Source: CAD feature listing. Evaluate the final solid. Frame: model axes, mm. Face numbers are marked on the shaded views. A direction names the side the tool comes from. Coordinates: 2 decimals unless noted, no trailing zeros. Write item = value, one per line. Start each with the question number.
1. Pull-direction query (Y, two-part tool) for the marked faces 1, 2 and 3; classes: pulls with the +Y half, pulls with the -Y half, needs draft (parallel to the pull), parting line crosses it, or undercut.
2. Pin query (flat end, axial travel): pin 1 Ø6 at (x, z) = (29.5, 2.5) entering from -Y; pin 2 Ø8 at (x, z) = (13, 4) entering from +Y; pin 3 Ø12 at (y, z) = (-34.5, 7) entering from -X. Return the tip coordinate at first contact, or that it passes through.
3. Section query A-A (z = 0.5). Give the number of separate pieces and of enclosed holes in the cut face, then the cut area to 3 significant figures.
4. Access query for the marked faces 4, 5 and 6. Directions: +Z, -Z, +X, -X, +Y, -Y. A direction counts if a zero-diameter tool reaches every point of the face in a straight line with its end or side. Return the directions, or none.
5. Line query: line 1 along X through (y, z) = (-36, 17.5); line 2 along X through (y, z) = (-38.5, 6.5); line 3 along Z through (x, y) = (10.5, 5.5). Output: solid intervals per line, ascending.
```python
from build123d import *

# Parameters (mm, degrees)
BOSS_EXTRUDE1_DEPTH      = 2
BOSS_EXTRUDE1_DEPTH_BACK = 7
BOSS_EXTRUDE3_DEPTH      = 9
SKETCH6_R                = 4
CUT_EXTRUDE1_DEPTH       = 18
BOSS_EXTRUDE4_DEPTH      = 18
SKETCH8_R                = 2.25
CUT_EXTRUDE2_DEPTH       = 69.863255609
CUT_EXTRUDE3_DEPTH       = 67.431528446
CUT_EXTRUDE3_DEPTH_BACK  = 67.431528446
SKETCH9_W                = 10.323299019
SKETCH9_H                = 27.481333942


with BuildPart() as part:
    # Sketch2 → Boss-Extrude1 (new, two sides: drawn at the far end of the back side and taken through both)
    with BuildSketch(Plane.XY.offset(-BOSS_EXTRUDE1_DEPTH_BACK)):
        with BuildLine():
            Line((17.593003447, 3.447921134), (18.432689254, 3.812129579))
            ThreePointArc((18.432689254, 3.812129579), (18.142308848, 4.822341152), (17.760116965, 5.801513031))
            Line((17.760116965, 5.801513031), (16.871688472, 5.581479263))
            Line((16.871688472, 5.581479263), (15.649099733, 5.241598415))
            ThreePointArc((15.649099733, 5.241598415), (15.22663553, 6.009376293), (14.733410626, 6.733729845))
            Line((14.733410626, 6.733729845), (15.590096731, 7.669855443))
            Line((15.590096731, 7.669855443), (16.188603379, 8.362321932))
            ThreePointArc((16.188603379, 8.362321932), (15.488665299, 9.146499772), (14.719475556, 9.862876308))
            Line((14.719475556, 9.862876308), (14.014498216, 9.279158058))
            Line((14.014498216, 9.279158058), (13.060452596, 8.442474621))
            ThreePointArc((13.060452596, 8.442474621), (12.346699165, 8.950918239), (11.588033655, 9.389535972))
            Line((11.588033655, 9.389535972), (11.95371149, 10.604658163))
            Line((11.95371149, 10.604658163), (12.192497398, 11.488231214))
            ThreePointArc((12.192497398, 11.488231214), (11.221632964, 11.891059284), (10.217792822, 12.202753318))
            Line((10.217792822, 12.202753318), (9.835896044, 11.370963143))
            Line((9.835896044, 11.370963143), (9.33935398, 10.203192533))
            ThreePointArc((9.33935398, 10.203192533), (8.475678941, 10.351598396), (7.601835833, 10.417606691))
            Line((7.601835833, 10.417606691), (7.404078418, 11.671055622))
            Line((7.404078418, 11.671055622), (7.235849109, 12.570732756))
            ThreePointArc((7.235849109, 12.570732756), (6.18634993, 12.512426015), (5.14668224, 12.357702722))
            Line((5.14668224, 12.357702722), (5.163505363, 11.442586867))
            Line((5.163505363, 11.442586867), (5.222813101, 10.175020376))
            ThreePointArc((5.222813101, 10.175020376), (4.380277888, 9.933994883), (3.564332526, 9.614319987))
            Line((3.564332526, 9.614319987), (2.842308143, 10.657834724))
            Line((2.842308143, 10.657834724), (2.300383494, 11.395423851))
            ThreePointArc((2.300383494, 11.395423851), (1.380115753, 10.887530665), (0.510539453, 10.297034891))
            Line((0.510539453, 10.297034891), (0.922750452, 9.479843274))
            Line((0.922750452, 9.479843274), (1.526161366, 8.363537991))
            ThreePointArc((1.526161366, 8.363537991), (0.871640411, 7.780819197), (0.275200782, 7.138776643))
            Line((0.275200782, 7.138776643), (-0.828084785, 7.765676295))
            Line((-0.828084785, 7.765676295), (-1.636369952, 8.195088843))
            ThreePointArc((-1.636369952, 8.195088843), (-2.245135941, 7.338203686), (-2.772390602, 6.42889036))
            Line((-2.772390602, 6.42889036), (-2.04643517, 5.871477804))
            Line((-2.04643517, 5.871477804), (-1.018434012, 5.12753168))
            ThreePointArc((-1.018434012, 5.12753168), (-1.355304806, 4.318534189), (-1.61410652, 3.481288379))
            Line((-1.61410652, 3.481288379), (-2.880134034, 3.567407782))
            Line((-2.880134034, 3.567407782), (-3.794688927, 3.603593329))
            ThreePointArc((-3.794688927, 3.603593329), (-3.971379595, 2.567432815), (-4.051883364, 1.519402593))
            Line((-4.051883364, 1.519402593), (-3.155967876, 1.332171491))
            Line((-3.155967876, 1.332171491), (-1.90698471, 1.107932181))
            ThreePointArc((-1.90698471, 1.107932181), (-1.859483953, 0.232887867), (-1.729388897, -0.633734398))
            Line((-1.729388897, -0.633734398), (-2.907406081, -1.105452248))
            Line((-2.907406081, -1.105452248), (-3.747091888, -1.469660694))
            ThreePointArc((-3.747091888, -1.469660694), (-3.456711482, -2.479872267), (-3.0745196, -3.459044145))
            Line((-3.0745196, -3.459044145), (-2.186091107, -3.239010378))
            Line((-2.186091107, -3.239010378), (-0.963502367, -2.899129529))
            ThreePointArc((-0.963502367, -2.899129529), (-0.541038164, -3.666907408), (-0.047813261, -4.391260959))
            Line((-0.047813261, -4.391260959), (-0.904499365, -5.327386558))
            Line((-0.904499365, -5.327386558), (-1.503006014, -6.019853046))
            ThreePointArc((-1.503006014, -6.019853046), (-0.803067933, -6.804030887), (-0.03387819, -7.520407423))
            Line((-0.03387819, -7.520407423), (0.67109915, -6.936689172))
            Line((0.67109915, -6.936689172), (1.625144769, -6.100005735))
            ThreePointArc((1.625144769, -6.100005735), (2.3388982, -6.608449353), (3.097563711, -7.047067087))
            Line((3.097563711, -7.047067087), (2.731885876, -8.262189278))
            Line((2.731885876, -8.262189278), (2.493099968, -9.145762328))
            ThreePointArc((2.493099968, -9.145762328), (3.463964401, -9.548590398), (4.467804544, -9.860284433))
            Line((4.467804544, -9.860284433), (4.849701322, -9.028494257))
            Line((4.849701322, -9.028494257), (5.346243386, -7.860723648))
            ThreePointArc((5.346243386, -7.860723648), (6.209918425, -8.009129511), (7.083761533, -8.075137806))
            Line((7.083761533, -8.075137806), (7.281518948, -9.328586736))
            Line((7.281518948, -9.328586736), (7.449748257, -10.22826387))
            ThreePointArc((7.449748257, -10.22826387), (8.499247436, -10.16995713), (9.538915126, -10.015233837))
            Line((9.538915126, -10.015233837), (9.522092003, -9.100117982))
            Line((9.522092003, -9.100117982), (9.462784265, -7.83255149))
            ThreePointArc((9.462784265, -7.83255149), (10.305319478, -7.591525998), (11.12126484, -7.271851101))
            Line((11.12126484, -7.271851101), (11.843289223, -8.315365839))
            Line((11.843289223, -8.315365839), (12.385213872, -9.052954966))
            ThreePointArc((12.385213872, -9.052954966), (13.305481612, -8.54506178), (14.175057913, -7.954566005))
            Line((14.175057913, -7.954566005), (13.762846914, -7.137374389))
            Line((13.762846914, -7.137374389), (13.159436, -6.021069105))
            ThreePointArc((13.159436, -6.021069105), (13.813956955, -5.438350311), (14.410396584, -4.796307757))
            Line((14.410396584, -4.796307757), (15.513682151, -5.42320741))
            Line((15.513682151, -5.42320741), (16.321967317, -5.852619957))
            ThreePointArc((16.321967317, -5.852619957), (16.930733307, -4.9957348), (17.457987967, -4.086421474))
            Line((17.457987967, -4.086421474), (16.732032536, -3.529008918))
            Line((16.732032536, -3.529008918), (15.704031377, -2.785062794))
            ThreePointArc((15.704031377, -2.785062794), (16.040902172, -1.976065303), (16.299703886, -1.138819493))
            Line((16.299703886, -1.138819493), (17.565731399, -1.224938896))
            Line((17.565731399, -1.224938896), (18.480286292, -1.261124443))
            ThreePointArc((18.480286292, -1.261124443), (18.656976961, -0.22496393), (18.737480729, 0.823066292))
            Line((18.737480729, 0.823066292), (17.841565242, 1.010297394))
            Line((17.841565242, 1.010297394), (16.592582076, 1.234536705))
            ThreePointArc((16.592582076, 1.234536705), (16.545081318, 2.109581019), (16.414986263, 2.976203284))
            Line((16.414986263, 2.976203284), (17.593003447, 3.447921134))
        make_face()
    extrude(amount=BOSS_EXTRUDE1_DEPTH + BOSS_EXTRUDE1_DEPTH_BACK)

    # Sketch5 → Boss-Extrude3 (add)
    with BuildSketch(Plane.XY.offset(2)):
        with BuildLine():
            Line((34.627961915, -50.407866333), (38.369192873, -48.55177457))
            Line((38.369192873, -48.55177457), (13.393984011, -14.920355903))
            Line((13.393984011, -14.920355903), (9.462784265, -7.83255149))
            Line((9.462784265, -7.83255149), (0.865656202, -2.843190202))
            Line((0.865656202, -2.843190202), (-0.03387819, -7.520407423))
            add(Edge.make_bspline(
                [(34.627961915, -50.407866333), (20.737528927, -38.343464696), (7.957182105, -24.264537371), (-0.03387819, -7.520407423)],
                knots=[0, 0, 0, 0, 1, 1, 1, 1], degree=3))
        make_face()
    extrude(amount=-BOSS_EXTRUDE3_DEPTH)

    # Sketch6 → Cut-Extrude1 (cut)
    with BuildSketch(Plane(origin=(0, 0, -7), x_dir=(-1, 0, 0), z_dir=(0, 0, -1))):
        with Locations((-7.342798683, 1.171234443)):
            Circle(SKETCH6_R)
    extrude(amount=-CUT_EXTRUDE1_DEPTH, mode=Mode.SUBTRACT)

    # Sketch7 → Boss-Extrude4 (add)
    with BuildSketch(Plane.XY.offset(2)):
        with BuildLine():
            Line((34.627961915, -50.407866333), (38.369192873, -48.55177457))
            Line((38.369192873, -48.55177457), (13.393984011, -14.920355903))
            add(Edge.make_bspline(
                [(7.977955023, -21.345123668), (8.112113434, -15.921271934), (13.393984011, -14.920355903)],
                knots=[0, 0, 0, 1, 1, 1], degree=2))
            add(Edge.make_bspline(
                [(7.977955023, -21.345123668), (15.413845314, -32.210109704), (24.739621619, -41.819443715), (34.627961915, -50.407866333)],
                knots=[0.288118642, 0.288118642, 0.288118642, 0.288118642, 1, 1, 1, 1], degree=3))
        make_face()
    extrude(amount=BOSS_EXTRUDE4_DEPTH)

    # Sketch8 → Cut-Extrude2 (cut, through all)
    with BuildSketch(Plane(origin=(0, 0, -7), x_dir=(-1, 0, 0), z_dir=(0, 0, -1))):
        with Locations((-14.312794722, -23.020807584)):
            Circle(SKETCH8_R)
        with Locations((-25.785580409, -37.215397344)):
            Circle(SKETCH8_R)
    extrude(amount=-CUT_EXTRUDE2_DEPTH, mode=Mode.SUBTRACT)

    # Sketch9 → Cut-Extrude3 (cut, two sides: drawn at the far end of the back side and taken through both)
    with BuildSketch(Plane(origin=(0, 0, 0), x_dir=(0, 0, -1), z_dir=(1, 0, 0)).offset(-CUT_EXTRUDE3_DEPTH_BACK)):
        with Locations((-4.16164951, 3.801629666)):
            Rectangle(SKETCH9_W, SKETCH9_H)
    extrude(amount=CUT_EXTRUDE3_DEPTH + CUT_EXTRUDE3_DEPTH_BACK, mode=Mode.SUBTRACT)


solid = part.part
```
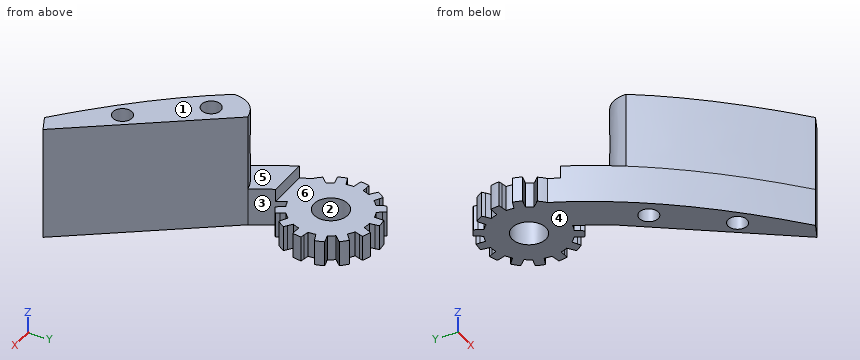
Results are:
q1.face_1 = needs draft
q1.face_2 = undercut
q1.face_3 = undercut
q2.pin_1 = -48.54
q2.pin_2 = -9.94
q2.pin_3 = 13.28
q3.separate_pieces = 1
q3.enclosed_holes = 2
q3.area = 330 mm^2
q4.face_4 = -Z, +X, -X, +Y, -Y
q4.face_5 = +Z, -X, +Y
q4.face_6 = +Z, +X, -X, +Y
q5.line_1 = 19.71 to 23.89, 27.68 to 29.05
q5.line_2 = 22.06 to 23.94, 27.63 to 30.9
q5.line_3 = -7 to -1
